Build history of the part. All positions in model axes, mm. Face numbers are marked on the shaded views. A direction names the side the tool comes from. Round coordinates to 2 decimals unless told otherwise and drop trailing zeros. Order: outer loops, then holes, each group sorted by start corner. A loop starts at its lowest first (then second) coordinate and runs counter-clockwise, first axis right, second up. Notation, with made-up numbers: (-17, 56.5) -> (5, 56.5) arc R27 ccw to (5, 92.5) -> close; hole circle Ø6 at (55.5, 73.25). An arc over 180 degrees is marked (long way). Answer as CSV lines item,"result". Start each with the question number.
```python
from build123d import *

# Parameters (mm, degrees)
ESQUISSE1_R        = 7
BOSS_EXTRU_1_DEPTH = 45


with BuildPart() as part:
    # Esquisse1 → Boss.-Extru.1 (new body)
    with BuildSketch(Plane.XY):
        with BuildLine():
            Line((0, 0), (29, 35))
            Line((29, 35), (29, 54))
            Line((29, 54), (24, 59))
            Line((24, 59), (0, 59))
            ThreePointArc((0, 59), (-8.408362672, 49.535902458), (-20.895957648, 47.455114912))
            Line((-20.895957648, 47.455114912), (-41, 51))
            Line((-41, 51), (-48, 51))
            Line((-48, 51), (-55, 44))
            Line((-55, 44), (-55, 26))
            Line((-55, 26), (-48, 19))
            Line((-48, 19), (-17.887486299, 19))
            ThreePointArc((-17.887486299, 19), (-14.622250518, 17.786586232), (-12.941847557, 14.735294118))
            ThreePointArc((-12.941847557, 14.735294118), (-10.605017354, 6.884327939), (-6.166045157, 0))
            Line((-6.166045157, 0), (0, 0))
        make_face()
        with Locations((-41, 33)):
            Circle(ESQUISSE1_R, mode=Mode.SUBTRACT)
    extrude(amount=-BOSS_EXTRU_1_DEPTH)


solid = part.part
```
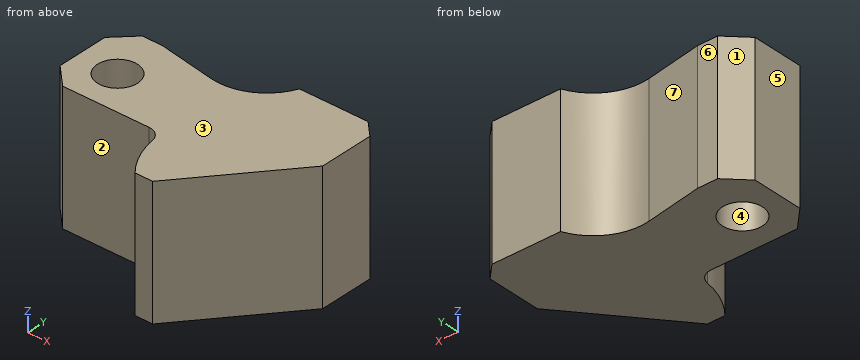
Q1. Slice it at B-B, the plane y = 33. Write the cut outline in (x, z).
Q2. Slice it at D-D, the plane y = 11. Write the cut outline in (x, z), plus the area to 3 significant figures.
Q3. Slice it at A-A, the plane z = -7.5. Write the cut outline in (x, y).
Q4. Flat gauge pins, fed straight in: pin 1 Ø1.5 at (x, z) = (-18.5, -27) entering from -Y; pin 2 Ø3 at (y, z) = (7.5, -35.5) entering from -X; pin 3 Ø8 at (x, z) = (17, -18.5) entering from -Y. Where does each tip first touch, or does it go through?
Q5. Probe L1, parallel to Y at x = -41, z = -21; L2, parallel to X at y = 35, z = -19; L3, parallel to Y at x = -0.5, z = -3. List the from-to ranges inside material, lowest first.
Q6. Slice it at C-C, the plane x = -15.5. Write the cut outline in (y, z).
Q7. Which spindle directions (+Z, -Z, +X, -X, +Y, -Y) get a long thin tool onto all of the face, cutting with end or side? Do the marked faces 5, 6 and 7. Say none if no direction does.
Q8. Two-plate mould, pull along Y, no slides. Class the marked faces 1, 2, 3 and 4: +Y half, -Y half, draft (parallel to the pull), parting line (faces both ways), or undercut.
Solutions:
1,outline,"(-55, -45) -> (-48, -45) -> (-48, 0) -> (-55, 0) -> close; (-34, -45) -> (27.34, -45) -> (27.34, 0) -> (-34, 0) -> close"
2,outline,"(-12.13, -45) -> (9.11, -45) -> (9.11, 0) -> (-12.13, 0) -> close"
2,area,"956 mm2"
3,outline,"(-55, 26) -> (-48, 19) -> (-17.89, 19) arc R5 cw to (-12.94, 14.74) arc R29 ccw to (-6.17, 0) -> (0, 0) -> (29, 35) -> (29, 54) -> (24, 59) -> (0, 59) arc R19 cw to (-20.9, 47.46) -> (-41, 51) -> (-48, 51) -> (-55, 44) -> close; hole circle Ø14 at (-41, 33)"
4,pin 1,"stops at y = 19"
4,pin 2,"stops at x = -11.48"
4,pin 3,"stops at y = 15.69"
5,L1,"y = 19 to 26, 40 to 51"
5,L2,"x = -55 to -47.71, -34.29 to 29"
5,L3,"y = 0 to 57.88"
6,outline,"(18.39, -45) -> (47.28, -45) -> (47.28, 0) -> (18.39, 0) -> close"
7,face 5,"+Z, -Z, -X, +Y, -Y"
7,face 6,"+Z, -Z, -X, +Y"
7,face 7,"+Z, -Z, +Y"
8,face 1,"+Y half"
8,face 2,"-Y half"
8,face 3,"draft"
8,face 4,"undercut"
